Work out the finished part from the listing and answer in its coordinate system (mm). Face numbers are marked on the shaded views. A direction names the side the tool comes from. Give positions to 0.01 mm unless a question says otherwise; leave off trailing zeros. Loops run counter-clockwise (first coordinate to the right, second up) from the corner with the lowest first, then second, coordinate; pieces in that order, holes last. Notation, with made-up numbers: M 15,73.25 L 42,73.25 A15 ccw 42,78.25 Z; hole C 43.25,80.5 d7. An arc over 180 degrees is marked long. Use a Markdown table: item, result.
Autodesk Inventor part; units mm, degrees
ref_plane "YZ Plane" through (0, 0, 0) normal (1, 0, 0) x (0, 1, 0)
ref_plane "XZ Plane" through (0, 0, 0) normal (0, 1, 0) x (-1, 0, 0)
ref_plane "XY Plane" through (0, 0, 0) normal (0, 0, 1) x (1, 0, 0)
sketch "Esquisse1" plane through (0, 0, 0) normal (0, 1, 0) x (-1, 0, 0)
  circle A0 centre (0, 0) radius 10.5
  circle A1 centre (0, 0) radius 12.5
  dimension "d0" = 21
  dimension "d1" = 25
extrude "Extrusion1" add sketch "Esquisse1" along normal blind 1
sketch "Esquisse2" plane through (0, 1, 0) normal (0, 1, 0) x (1, 0, 0)
  circle A0 centre (0, 0) radius 12.5
  circle A1 centre (0, 0) radius 11.5
  dimension "d4" = 23
  dimension "d5" = 25
extrude "Extrusion2" add sketch "Esquisse2" along normal blind 12
sketch "Esquisse3" plane through (0, 13, 0) normal (0, 1, 0) x (1, 0, 0)
  line L0 (-5, -12.5) -> (5, -12.5)
  line L1 (5, -12.5) -> (5, -10.3562)
  line L2 (5, 12.5) -> (-5, 12.5)
  line L3 (-5, 12.5) -> (-5, 10.3562)
  circle A0 centre (0, 0) radius 12.5
  arc A1 (-5, 10.3562) -> (-5, -10.3562) centre (0, 0) ccw
  circle A2 centre (0, 0) radius 11.5
  arc A3 (5, 10.3562) -> (-5, 10.3562) centre (0, 0) ccw
  arc A4 (-5, -10.3562) -> (5, -10.3562) centre (0, 0) ccw
  arc A5 (5, -10.3562) -> (5, 10.3562) centre (0, 0) ccw
  line L4 (-5, 10.3562) -> (-5, -10.3562)
  line L5 (-5, -10.3562) -> (-5, -12.5)
  line L6 (5, 10.3562) -> (5, 12.5)
  line L7 (5, -10.3562) -> (5, 10.3562)
  dimension "d8" = 5
  dimension "d9" = 5
  dimension "d10" = 0
extrude "Extrusion3" add sketch "Esquisse3" against normal blind 5 contours L5 A0 L0 | A0 L1 L0 | A0 L5 A2 L1 | A0 L6 A2 L3 | L3 L2 A0 | L2 L6 A0
sketch "Esquisse4" plane through (-5, 13, 12.5) normal (0, 0, 1) x (1, 0, 0)
  line L0 (10, -5) -> (0, 0) construction
  line L1 (10, 0) -> (0, -5) construction
  circle A0 centre (5, -2.5) radius 1.75
  point P0 (5, -13)
  dimension "d13" = 3.5
extrude "Extrusion4" cut sketch "Esquisse4" against normal through all
sketch "Esquisse6" plane through (0, 13, 0) normal (0, 1, 0) x (1, 0, 0)
  line L0 (-12.5, -2) -> (12.5, -2)
  line L1 (12.5, -2) -> (12.5, 2)
  line L2 (12.5, 2) -> (-12.5, 2)
  line L3 (-12.5, 2) -> (-12.5, -2)
  arc A0 (-5, 11.4564) -> (-5, -11.4564) centre (0, 0) ccw
  arc A1 (5, -11.4564) -> (5, 11.4564) centre (0, 0) ccw
  dimension "d17" = 4
  dimension "d18" = 2
extrude "Extrusion5" cut sketch "Esquisse6" against normal blind 9.5
sketch "Esquisse7" plane through (0, 3.5, 0) normal (0, 1, 0) x (1, 0, 0)
  line L0 (-12.5, -2) -> (12.5, -2)
  line L1 (12.5, -2) -> (12.5, 0)
  line L2 (12.5, 2) -> (-12.5, 2)
  line L3 (-12.5, 2) -> (-12.5, 0)
  line L4 (-11.3248, -2) -> (-12.339, -2)
  line L5 (-12.339, 2) -> (-11.3248, 2)
  arc A0 (-12.339, 2) -> (-12.339, -2) centre (0, 0) ccw
  arc A1 (12.339, -2) -> (12.339, 2) centre (0, 0) ccw
  line L6 (-12.5, 0) -> (12.5, 0)
  line L7 (-12.5, 0) -> (-12.5, -2)
  line L8 (12.5, 0) -> (12.5, 2)
revolve "Révolution1" cut sketch "Esquisse7" angle 360 about axis through (-12.5, 3.5, 0) along (1, 0, 0) contours L3 L2 A0 | A0 L2 A1 L6 | A1 L2 L8
equation "\"d18\" = 0.5 * d17"
properties part number "optoforce_base"
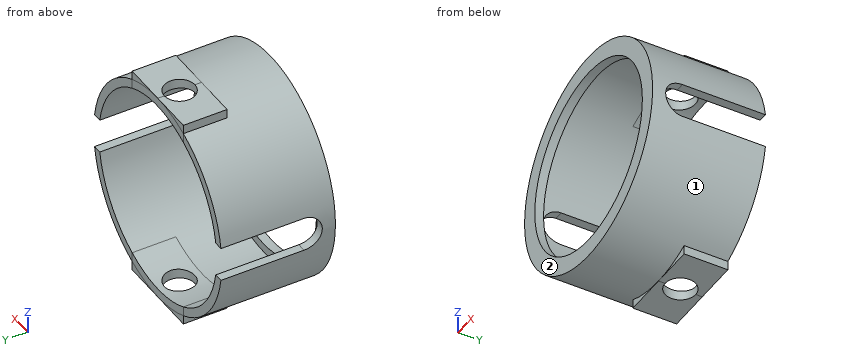
(1) Given P1, Ø0.8, axis at x = -12, y = 7, coming from the -Z side; P2, Ø0.8, axis at y = 10.5, z = -12, coming from the -X side; P3, Ø0.8, axis at y = 11, z = 12, coming from the +X side; P4, Ø14, axis at x = 0, z = 0, coming from the +Y side, each flat-ended and moving along its own axis, determine where each tip first touches the part or whether it passes through.
Entries:
| item | result |
|---|---|
| P1 | stops at z = -4.66 |
| P2 | stops at x = -5 |
| P3 | stops at x = 5 |
| P4 | passes through |
(2) A cutting plane is placed at C-C (z = -7). Write down the section's boundary in (x, y).
Entries:
| item | result |
|---|---|
| outline | M -10.36,0 L -7.83,0 L -7.83,1 L -9.12,1 L -9.12,13 L -10.36,13 Z; M 7.83,0 L 10.36,0 L 10.36,13 L 9.12,13 L 9.12,1 L 7.83,1 Z |
(3) Which of the six approach directions +Z, -Z, +X, -X, +Y, -Y give full straight-line access (tool end or side, diameter ignored) to the marked faces 1 and 2?
Entries:
| item | result |
|---|---|
| face 1 | -Y |
| face 2 | +Z, -Z, +X, -X, -Y |
(4) A cutting plane is placed at B-B (y = 4). Write down the section's boundary in (x, z), and give its area (3 significant figures).
Entries:
| item | result |
|---|---|
| outline | M -12.34,-2 A12.5 ccw 12.34,-2 L 11.32,-2 A11.5 cw -11.32,-2 Z; M -12.34,2 L -11.32,2 A11.5 cw 11.32,2 L 12.34,2 A12.5 ccw Z |
| area | 67.4 mm² |
(5) A cutting plane is placed at A-A (y = 10.5). Write down the section's boundary in (x, z), and give its area (3 significant figures).
Entries:
| item | result |
|---|---|
| outline | M -12.34,-2 A12.5 ccw -5,-11.46 L -5,-12.5 L -1.75,-12.5 L -1.75,-11.37 A11.5 cw -11.32,-2 Z; M -12.34,2 L -11.32,2 A11.5 cw -1.75,11.37 L -1.75,12.5 L -5,12.5 L -5,11.46 A12.5 ccw Z; M 1.75,-12.5 L 5,-12.5 L 5,-11.46 A12.5 ccw 12.34,-2 L 11.32,-2 A11.5 cw 1.75,-11.37 Z; M 1.75,11.37 A11.5 cw 11.32,2 L 12.34,2 A12.5 ccw 5,11.46 L 5,12.5 L 1.75,12.5 Z |
| area | 66.9 mm² |
(6) Consider probe 1 along X at (y, z) = (10.5, 12); probe 2 along Z at (x, y) = (0, 0.55); probe 3 along Y at (x, z) = (0, -11.7). Determine where each line is inside the solid, lowest interval first. Write a range as [from, to].
Entries:
| item | result |
|---|---|
| probe 1 | x = [-5, -1.75], [1.75, 5] |
| probe 2 | z = [-12.5, -10.5], [10.5, 12.5] |
| probe 3 | y = [0, 8.75], [12.25, 13] |
